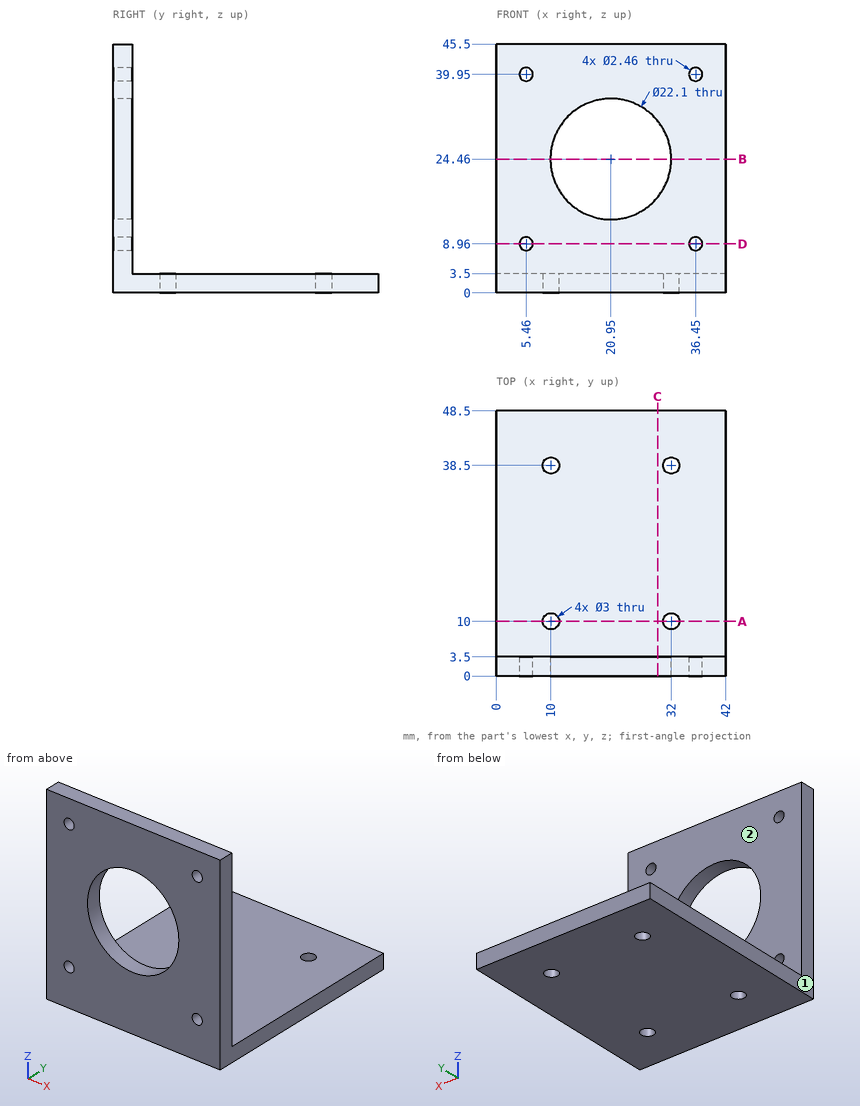
Print and shaded views of the part. All mm, measured from the part's lowest x, y and z. A direction names the side the tool comes from. Give positions to 0.01 mm unless a question says otherwise; leave off trailing zeros. Loops run counter-clockwise (first coordinate to the right, second up) from the corner with the lowest first, then second, coordinate; pieces in that order, holes last. Notation, with made-up numbers: (-28.75, 42.25) - (16.25, 42.25) arc R12 ccw to (16.25, 59.25) - close; hole circle Ø3 at (-27.5, -24). An arc over 180 degrees is marked (long way). Use a Markdown table: item, result.
(1) Band-saw the part on D-D (z = 8.96). Give the cut face in (x, y), and give its area (3 significant figures).
Taken from the geometry:
| item | result |
|---|---|
| outline | (0, 0) - (4.23, 0) - (4.23, 3.5) - (0, 3.5) - close; (6.69, 0) - (35.22, 0) - (35.22, 3.5) - (6.69, 3.5) - close; (37.68, 0) - (42, 0) - (42, 3.5) - (37.68, 3.5) - close |
| area | 130 mm2 |
(2) Drop flat-ended pins along their axis: pin 1 Ø4 at (x, y) = (10, 10) entering from +Z; pin 2 Ø2.5 at (x, y) = (32, 38.5) entering from +Z; pin 3 Ø1.5 at (x, z) = (27.5, 14.5) entering from +Y. Give the stop position or say it passes through.
Taken from the geometry:
| item | result |
|---|---|
| pin 1 | z = 3.5 |
| pin 2 | through |
| pin 3 | y = 3.5 |
(3) Band-saw the part on A-A (y = 10). Give the cut face in (x, z).
Taken from the geometry:
| item | result |
|---|---|
| outline | (0, 0) - (8.5, 0) - (8.5, 3.5) - (0, 3.5) - close; (11.5, 0) - (30.5, 0) - (30.5, 3.5) - (11.5, 3.5) - close; (33.5, 0) - (42, 0) - (42, 3.5) - (33.5, 3.5) - close |
(4) Band-saw the part on C-C (x = 29.5). Give the cut face in (y, z).
Taken from the geometry:
| item | result |
|---|---|
| outline | (0, 0) - (48.5, 0) - (48.5, 3.5) - (3.5, 3.5) - (3.5, 17.46) - (0, 17.46) - close; (0, 31.46) - (3.5, 31.46) - (3.5, 45.5) - (0, 45.5) - close |
(5) Which spindle directions (+Z, -Z, +X, -X, +Y, -Y) get a long thin tool onto all of the face, cutting with end or side? Do the marked faces 1 and 2. Say none if no direction does.
Taken from the geometry:
| item | result |
|---|---|
| face 1 | +Z, -Z, -X, +Y, -Y |
| face 2 | +Z, +X, -X, +Y |
(6) Wall check: line 1 along Y through (x, z) = (10, 1); line 2 along Z through (x, y) = (6, 34.5); line 3 along X through (y, z) = (1, 39). Give the ranges that are in metal, low to high.
Taken from the geometry:
| item | result |
|---|---|
| line 1 | 0 to 8.5, 11.5 to 37, 40 to 48.5 |
| line 2 | 0 to 3.5 |
| line 3 | 0 to 4.68, 6.24 to 35.67, 37.23 to 42 |
(7) Band-saw the part on B-B (z = 24.46). Give the cut face in (x, y), and give its area (4 significant figures).
Taken from the geometry:
| item | result |
|---|---|
| outline | (0, 0) - (9.9, 0) - (9.9, 3.5) - (0, 3.5) - close; (32, 0) - (42, 0) - (42, 3.5) - (32, 3.5) - close |
| area | 69.65 mm2 |
